Part model, mm, in its own coordinate system. Face numbers are marked on the shaded views. Coordinates: 2 decimals unless noted, no trailing zeros. Write each loop counter-clockwise with the first axis right and the second up, starting at its lowest first coordinate (ties: lowest second). Pieces come first, ordered by that corner, then holes. Notation, with made-up numbers: (54, 17.5) - (74, 17.5) arc R20 ccw to (74, 25.5) - close; hole circle Ø6 at (46.5, 48.25). An arc over 180 degrees is marked (long way). Use a Markdown table: item, result.
Autodesk Inventor part; units mm, degrees
ref_plane "YZ Plane" through (0, 0, 0) normal (1, 0, 0) x (0, 1, 0)
ref_plane "XZ Plane" through (0, 0, 0) normal (0, 1, 0) x (-1, 0, 0)
ref_plane "XY Plane" through (0, 0, 0) normal (0, 0, 1) x (1, 0, 0)
sketch "スケッチ1" plane through (0, 0, 0) normal (1, 0, 0) x (0, 1, 0)
  line L0 (7, 0) -> (7, 0)
  line L1 (0, -9) -> (0, -14)
  line L2 (0, -14) -> (27, -14)
  line L3 (27, -14) -> (27, -11)
  line L4 (27, -11) -> (25, -11)
  line L5 (25, -11) -> (25, 0)
  line L6 (25, 0) -> (7, 0)
  line L7 (7, 0) -> (4, 0)
  line L8 (4, 0) -> (4, -9)
  line L9 (4, -9) -> (0, -9)
  point P0 (0, 0)
  dimension "d2" = 11
  dimension "d3" = 3
  dimension "d4" = 25
  dimension "d5" = 2
  dimension "d35" = 0
  dimension "d36" = 7
  dimension "d37" = 4
  dimension "d45" = 9
revolve "回転1" add sketch "スケッチ1" angle 360 about axis through (0, 0, -9) along (0, 0, -1)
chamfer "面取り1" distance 1 angle 45 1 edges at (0, -25, 0)
sketch "スケッチ2" plane through (0, 0, -14) normal (0, 0, -1) x (-1, 0, 0)
  point P0 (0, 0)
hole "穴1" at (0, 0, -14) direction (0, 0, 1) diameter 4.5 end through all
sketch "スケッチ3" plane through (0, 0, -14) normal (0, 0, -1) x (-1, 0, 0)
  circle A0 centre (0, 0) radius 21
  point P0 (0, 0)
  point P1 (0, -21)
  point P2 (18.1865, -10.5)
  point P3 (18.1865, 10.5)
  point P4 (0, 21)
  point P5 (-18.1865, 10.5)
  point P6 (-18.1865, -10.5)
  dimension "d20" = 42
  dimension "d23" = 360
hole "穴2" at (0, -21, -14) at (-18.1865, -10.5, -14) at (-18.1865, 10.5, -14) at (0, 21, -14) at (18.1865, 10.5, -14) at (18.1865, -10.5, -14) direction (0, 0, 1) diameter 3.2 end through all
chamfer "面取り4" distance 0.5 angle 45 1 edges at (0, -4, 0)
properties part number "base3" material "ABS プラスチック"
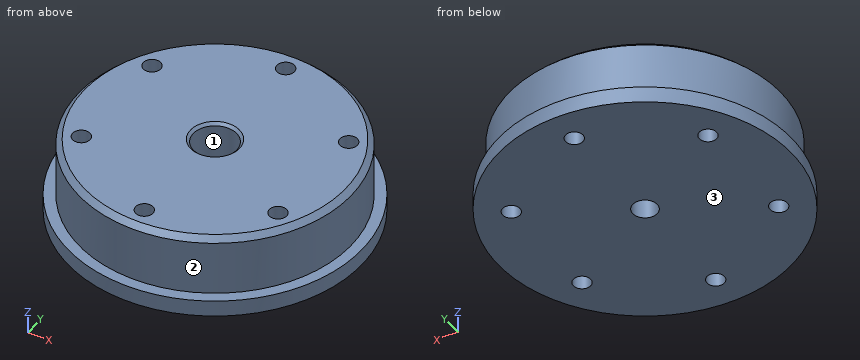
Item 1: Drill centre lines: probe 1 along X at (y, z) = (0, -11.4); probe 2 along X at (y, z) = (10.5, -9); probe 3 along Y at (x, z) = (1, -13). Where is each one in solid material? Low to high.
From the geometry:
| item | result |
|---|---|
| probe 1 | -27 to -2.25, 2.25 to 27 |
| probe 2 | -22.69 to -19.79, -16.59 to 16.59, 19.79 to 22.69 |
| probe 3 | -26.98 to -22.25, -19.75 to -2.02, 2.02 to 19.75, 22.25 to 26.98 |
Item 2: Band-saw the part on A-A, the plane y = 0. Give the cut face in (x, z), then the cut area to 3 significant figures.
From the geometry:
| item | result |
|---|---|
| outline | (-27, -14) - (-2.25, -14) - (-2.25, -9) - (-4, -9) - (-4, -0.5) - (-4.5, 0) - (-24, 0) - (-25, -1) - (-25, -11) - (-27, -11) - close; (2.25, -14) - (27, -14) - (27, -11) - (25, -11) - (25, -1) - (24, 0) - (4.5, 0) - (4, -0.5) - (4, -9) - (2.25, -9) - close |
| area | 616 mm^2 |
Item 3: Band-saw the part on C-C, the plane z = -10.25. Give the cut face in (x, y), then the cut area to 3 significant figures.
From the geometry:
| item | result |
|---|---|
| outline | circle Ø50 at (0, 0); hole circle Ø3.2 at (-18.19, -10.5); hole circle Ø3.2 at (-18.19, 10.5); hole circle Ø4.5 at (0, 0); hole circle Ø3.2 at (0, -21); hole circle Ø3.2 at (0, 21); hole circle Ø3.2 at (18.19, -10.5); hole circle Ø3.2 at (18.19, 10.5) |
| area | 1,900 mm^2 |
Item 4: Drop flat-ended pins along their axis: P1, Ø6, axis at x = 4, z = -6, coming from the +Y side; P2, Ø6, axis at y = 13, z = -8.5, coming from the +X side; P3, Ø6.5, axis at x = 0, y = 0, coming from the +Z side. Give the stop position or say it passes through.
From the geometry:
| item | result |
|---|---|
| P1 | y = 24.98 |
| P2 | x = 24.5 |
| P3 | z = -9 |
Item 5: Band-saw the part on B-B, the plane x = 0. Give the cut face in (y, z), then the cut area to 3 significant figures.
From the geometry:
| item | result |
|---|---|
| outline | (-27, -14) - (-22.6, -14) - (-22.6, 0) - (-24, 0) - (-25, -1) - (-25, -11) - (-27, -11) - close; (-19.4, -14) - (-2.25, -14) - (-2.25, -9) - (-4, -9) - (-4, -0.5) - (-4.5, 0) - (-19.4, 0) - close; (2.25, -14) - (19.4, -14) - (19.4, 0) - (4.5, 0) - (4, -0.5) - (4, -9) - (2.25, -9) - close; (22.6, -14) - (27, -14) - (27, -11) - (25, -11) - (25, -1) - (24, 0) - (22.6, 0) - close |
| area | 527 mm^2 |
Item 6: Two-plate mould, pull along Y, no slides. Class the marked faces 1, 2 and 3: pulls with the +Y half, pulls with the -Y half, needs draft (parallel to the pull), parting line crosses it, or undercut.
From the geometry:
| item | result |
|---|---|
| face 1 | undercut |
| face 2 | parting line crosses it |
| face 3 | needs draft |
Item 7: Band-saw the part on D-D, the plane y = 10.5. Count the separate pieces of the cut face and the enclosed holes in it, then the cut area to 3 significant figures.
From the geometry:
| item | result |
|---|---|
| separate pieces | 3 |
| enclosed holes | 0 |
| area | 558 mm^2 |
